Work out the finished part from the listing and answer in its coordinate system (mm). A direction names the side the tool comes from. Coordinates: 2 decimals unless noted, no trailing zeros. Loops run counter-clockwise (first coordinate to the right, second up) from the corner with the lowest first, then second, coordinate; pieces in that order, holes last. Notation, with made-up numbers: (52, -30) -> (91, -30) arc R17 cw to (91, -5) -> close; hole circle Ø1 at (-28.5, 52). An arc over 180 degrees is marked (long way). Use a Markdown table: item, result.
from build123d import *

# Parameters (mm, degrees)
SKETCH_1_R          = 15
EXTRUDE_1_DEPTH     = 10
SKETCH_2_R          = 7.5
EXTRUDE_2_DEPTH     = 5
CUT_EXTRUDE_1_DEPTH = 5
SKETCH_4_R          = 2.7
CUT_EXTRUDE_2_DEPTH = 5
SKETCH_5_R          = 1.05
CUT_EXTRUDE_3_DEPTH = 24.452078799
SKETCH_6_W          = 3.1
SKETCH_6_H          = 14.99101371
CUT_EXTRUDE_4_DEPTH = 8


with BuildPart() as part:
    # 草图1 → 凸台-拉伸1 (new body)
    with BuildSketch(Plane(origin=(0, 0, 0), x_dir=(0, 0, -1), z_dir=(1, 0, 0))):
        Circle(SKETCH_1_R)
    extrude(amount=EXTRUDE_1_DEPTH)

    # 草图2 → 凸台-拉伸2 (add)
    with BuildSketch(Plane(origin=(10, 0, 0), x_dir=(0, 0, -1), z_dir=(1, 0, 0))):
        Circle(SKETCH_2_R)
    extrude(amount=EXTRUDE_2_DEPTH)

    # 草图3 → 切除-拉伸1 (cut)
    with BuildSketch(Plane(origin=(15, 0, 0), x_dir=(0, 0, -1), z_dir=(1, 0, 0))):
        with BuildLine():
            Line((-2.025561651, 1.86), (2.025561651, 1.86))
            ThreePointArc((2.025561651, 1.86), (2.75, 0), (2.025561651, -1.86))
            Line((2.025561651, -1.86), (-2.025561651, -1.86))
            ThreePointArc((-2.025561651, -1.86), (-2.75, 0), (-2.025561651, 1.86))
        make_face()
    extrude(amount=-CUT_EXTRUDE_1_DEPTH, mode=Mode.SUBTRACT)

    # 草图4 → 切除-拉伸2 (cut)
    with BuildSketch(Plane.ZY):
        Circle(SKETCH_4_R)
    extrude(amount=-CUT_EXTRUDE_2_DEPTH, mode=Mode.SUBTRACT)

    # 草图5 → 切除-拉伸3 (cut, through all)
    with BuildSketch(Plane.ZY.offset(-5)):
        Circle(SKETCH_5_R)
    extrude(amount=-CUT_EXTRUDE_3_DEPTH, mode=Mode.SUBTRACT)

    # 草图6 → 切除-拉伸4 (cut)
    with BuildSketch(Plane.ZY):
        Polygon((18.533607515, 7.651700572), (19.491560198, 4.703425371), (5.234258923, 0.070947372), (4.27630624, 3.019222572), align=None)
        with Locations((0, 12.495506855)):
            Rectangle(SKETCH_6_W, SKETCH_6_H)
        Polygon((13.004399379, -15.262002685), (10.496446696, -17.084136968), (1.68494992, -4.956152113), (4.192902603, -3.134017831), align=None)
        Polygon((-10.496446696, -17.084136968), (-13.004399379, -15.262002685), (-4.192902603, -3.134017831), (-1.68494992, -4.956152113), align=None)
        Polygon((-19.491560198, 4.703425371), (-18.533607515, 7.651700572), (-4.27630624, 3.019222572), (-5.234258923, 0.070947372), align=None)
    extrude(amount=-CUT_EXTRUDE_4_DEPTH, mode=Mode.SUBTRACT)


solid = part.part
Q1. Section D-D on z = 12.25 is taken. Determine the outline of the cut face in (x, y).
Solved:
| item | result |
|---|---|
| outline | (0, -8.66) -> (10, -8.66) -> (10, 8.66) -> (0, 8.66) -> (0, 5.61) -> (8, 5.61) -> (8, 2.35) -> (0, 2.35) -> close |
Q2. Section A-A on x = 6 is taken. Determine the outline of the cut face in (y, z).
Solved:
| item | result |
|---|---|
| outline | (-12.98, -7.52) -> (-4.96, -1.68) -> (-3.13, -4.19) -> (-11.16, -10.02) arc R15 ccw to (3.14, -14.67) -> (0.07, -5.23) -> (3.02, -4.28) -> (6.08, -13.71) arc R15 ccw to (14.92, -1.55) -> (5, -1.55) -> (5, 1.55) -> (14.92, 1.55) arc R15 ccw to (6.08, 13.71) -> (3.02, 4.28) -> (0.07, 5.23) -> (3.14, 14.67) arc R15 ccw to (-11.16, 10.02) -> (-3.13, 4.19) -> (-4.96, 1.68) -> (-12.98, 7.52) arc R15 ccw to start; hole circle Ø2.1 at (0, 0) |
Q3. Section C-C on y = 12 is taken. Determine the outline of the cut face in (x, z), and give its area (3 significant figures).
Solved:
| item | result |
|---|---|
| outline | (0, -9) -> (10, -9) -> (10, 9) -> (0, 9) -> (0, 1.55) -> (8, 1.55) -> (8, -1.55) -> (0, -1.55) -> close |
| area | 155 mm² |
Q4. Consider line 1 (Y direction, x = 2.7, z = 0); line 2 (Y direction, x = 7.3, z = 0); line 3 (Z direction, x = 5.5, y = -8.25). Determine where each line is inside the solid, lowest interval first. Write a range as [from, to].
Solved:
| item | result |
|---|---|
| line 1 | [-15, -2.7], [2.7, 5] |
| line 2 | [-15, -1.05], [1.05, 5] |
| line 3 | [-12.53, -7.91], [-4.08, 4.08], [7.91, 12.53] |
Q5. Given pin 1 Ø2.5 at (x, y) = (3.5, 7.5) entering from -Z; pin 2 Ø1.2 at (x, z) = (12.5, 0.5) entering from +Y; pin 3 Ø1.9 at (y, z) = (-0.5, 0) entering from +X, each flat-ended and moving along its own axis, determine where each tip first touches the part or whether it passes through.
Solved:
| item | result |
|---|---|
| pin 1 | z = -13.64 |
| pin 2 | y = 7.5 |
| pin 3 | x = 10 |
Q6. Section B-B on z = 0 is taken. Determine the outline of the cut face in (x, y).
Solved:
| item | result |
|---|---|
| outline | (0, -15) -> (10, -15) -> (10, -7.5) -> (15, -7.5) -> (15, -1.86) -> (10, -1.86) -> (10, -1.05) -> (5, -1.05) -> (5, -2.7) -> (0, -2.7) -> close; (0, 2.7) -> (5, 2.7) -> (5, 1.05) -> (10, 1.05) -> (10, 1.86) -> (15, 1.86) -> (15, 7.5) -> (10, 7.5) -> (10, 15) -> (8, 15) -> (8, 5) -> (0, 5) -> close |
Q7. For faces 1 (the flat face through (15, 0, -3)), 2 (the cylindrical face through (2.465, -2.636, -0.585)), 3 (the flat face through (13, -1.86, 0)), 4 (the flat face through (4, 10, 1.55)), determine the directions among +Z, -Z, +X, -X, +Y, -Y from which every point of the face is accessible in a straight line to the end or side of a thin tool.
Solved:
| item | result |
|---|---|
| face 1 | +Z, -Z, +X, +Y, -Y |
| face 2 | -X |
| face 3 | +X |
| face 4 | -X, +Y |
